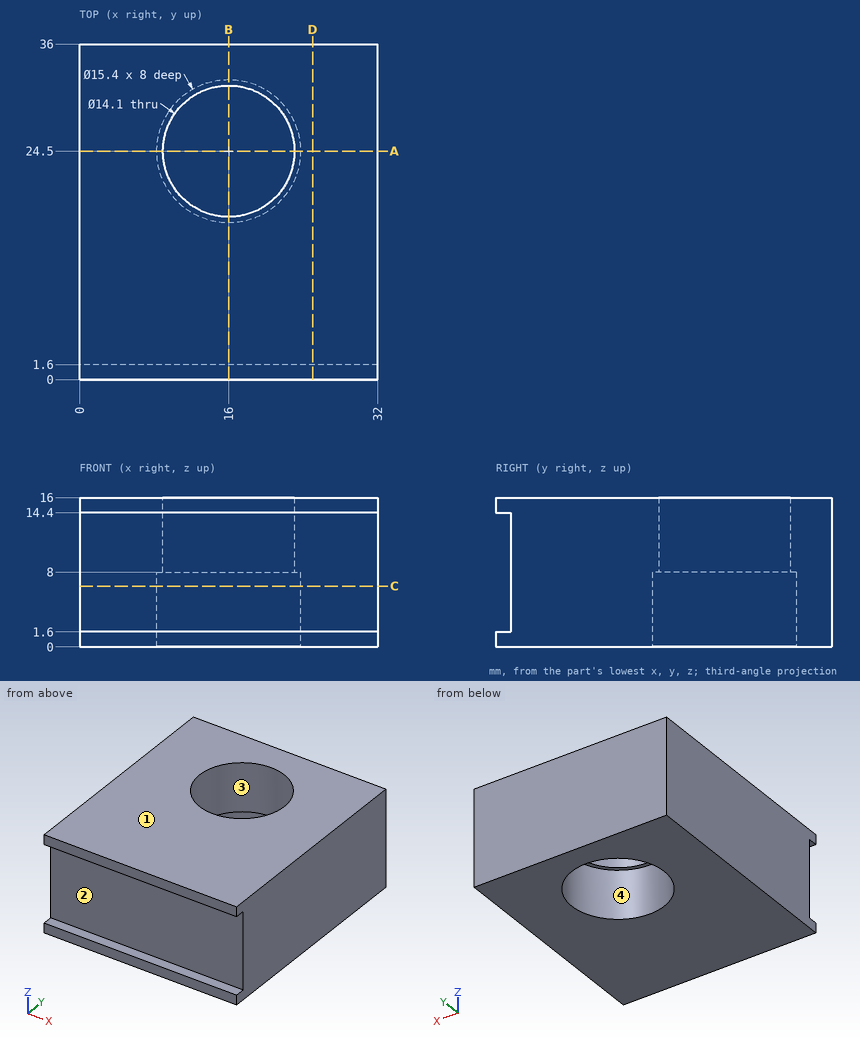
Geometry: see drawing. Coordinates: mm, zero at the bounding-box minimum. Coordinates: 2 decimals unless noted, no trailing zeros. Loops run counter-clockwise (first coordinate to the right, second up) from the corner with the lowest first, then second, coordinate; pieces in that order, holes last.
(1) Material intervals for probe 1 along Y at (x, z) = (16, 13); probe 2 along Y at (x, z) = (16, 6.25); probe 3 along Y at (x, z) = (2, 12), sorted ascending.
(2) Section C-C on z = 6.5. Return the cut outline in (x, y), then the cut area to 3 significant figures.
(3) Pull-direction query (Y, two-part tool) for the marked faces 1, 2, 3 and 4; classes: released by +Y, released by -Y, zero draft, split by the parting line, or undercut.
(4) First-contact query: pin 1 Ø4 at (x, z) = (22, 9.5) entering from -Y; pin 2 Ø12.5 at (x, y) = (16, 24.5) entering from -Z. Flat tips, straight axial feed; report the tip coordinate or a pass-through.
(5) Section D-D on x = 25. Return the cut outline in (y, z), then the cut area to 3 significant figures.
(6) Section A-A on y = 24.5. Return the cut outline in (x, z), then the cut area to 3 significant figures.
(7) Section B-B on x = 16. Return the cut outline in (y, z).
Data:
1. probe 1: y = 1.6 to 17.45, 31.55 to 36
1. probe 2: y = 1.6 to 16.8, 32.2 to 36
1. probe 3: y = 1.6 to 36
2. outline: (0, 1.6) - (32, 1.6) - (32, 36) - (0, 36) - close; hole circle Ø15.4 at (16, 24.5)
2. area: 915 mm2
3. face 1: zero draft
3. face 2: released by -Y
3. face 3: undercut
3. face 4: undercut
4. pin 1: stops at y = 1.6
4. pin 2: passes through
5. outline: (0, 0) - (36, 0) - (36, 16) - (0, 16) - (0, 14.4) - (1.6, 14.4) - (1.6, 1.6) - (0, 1.6) - close
5. area: 556 mm2
6. outline: (0, 0) - (8.3, 0) - (8.3, 8) - (8.95, 8) - (8.95, 16) - (0, 16) - close; (23.05, 8) - (23.7, 8) - (23.7, 0) - (32, 0) - (32, 16) - (23.05, 16) - close
6. area: 276 mm2
7. outline: (0, 0) - (16.8, 0) - (16.8, 8) - (17.45, 8) - (17.45, 16) - (0, 16) - (0, 14.4) - (1.6, 14.4) - (1.6, 1.6) - (0, 1.6) - close; (31.55, 8) - (32.2, 8) - (32.2, 0) - (36, 0) - (36, 16) - (31.55, 16) - close
